Design review of the part shown in the three views and the two pictorial views. Dimensions are in mm from the part's minimum x, y and z. Coordinates: 2 decimals unless noted, no trailing zeros. Loops run counter-clockwise (first coordinate to the right, second up) from the corner with the lowest first, then second, coordinate; pieces in that order, holes last. Notation, with made-up numbers: (55, -33) -> (88, -33) arc R18 ccw to (88, -18) -> close; hole circle Ø8 at (25, -40). An arc over 180 degrees is marked (long way). Answer in a Markdown table with one row per item.
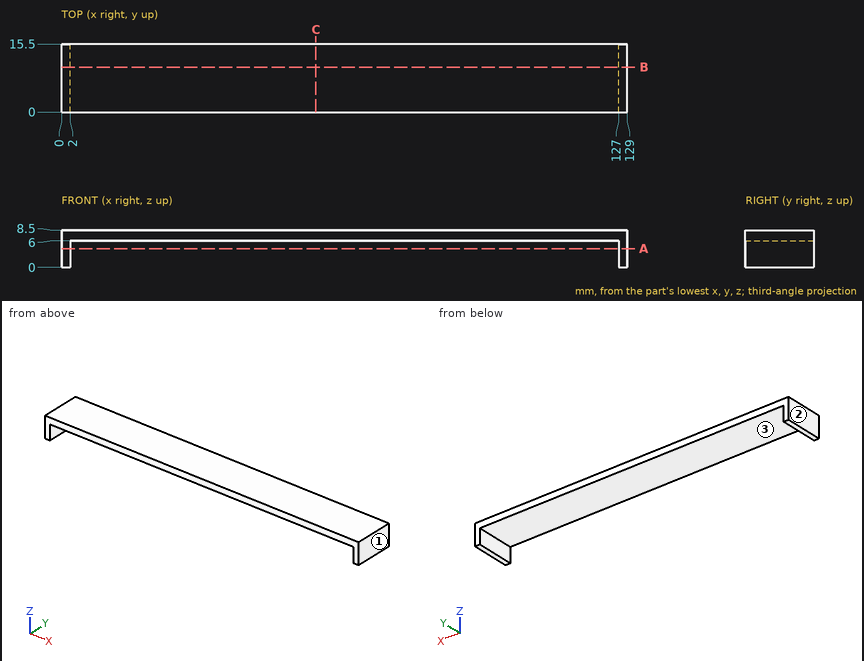
Item 1: For L1, parallel to X at y = 7.5, z = 4; L2, parallel to Z at x = 40, y = 13.75, list the stretches that pass through material, from the lowest coordinate up.
Worked answers:
| item | result |
|---|---|
| L1 | 0 to 2, 127 to 129 |
| L2 | 6 to 8.5 |
Item 2: Take a section at A-A, the plane z = 4.25. State the section outline as (x, y) points, and give its area (3 significant figures).
Worked answers:
| item | result |
|---|---|
| outline | (0, 0) -> (2, 0) -> (2, 15.5) -> (0, 15.5) -> close; (127, 0) -> (129, 0) -> (129, 15.5) -> (127, 15.5) -> close |
| area | 62.0 mm² |
Item 3: Take a section at C-C, the plane x = 58. State the section outline as (y, z) points.
Worked answers:
| item | result |
|---|---|
| outline | (0, 6) -> (15.5, 6) -> (15.5, 8.5) -> (0, 8.5) -> close |
Item 4: The part is to be moulded in two halves that separate along X. For the marked faces 1, 2 and 3, say which applies: +X half, -X half, draft (parallel to the pull), parting line (faces both ways), or undercut.
Worked answers:
| item | result |
|---|---|
| face 1 | +X half |
| face 2 | -X half |
| face 3 | undercut |
Item 5: Take a section at B-B, the plane y = 10.25. State the section outline as (x, z) points.
Worked answers:
| item | result |
|---|---|
| outline | (0, 0) -> (2, 0) -> (2, 6) -> (127, 6) -> (127, 0) -> (129, 0) -> (129, 8.5) -> (0, 8.5) -> close |
Item 6: Insertion check: pin 1 (1.8 mm diameter, centred on y = 6, z = 2, fed in from -X); pin 2 (2 mm diameter, centred on x = 113, y = 1.5, fed in from -Z). Each pin has a flat end and moves straight along its axis. Give the tip position at first contact, or say it passes through.
Worked answers:
| item | result |
|---|---|
| pin 1 | x = 0 |
| pin 2 | z = 6 |
